```python
from build123d import *

# Parameters (mm, degrees)
SKETCH2_3_R             = 1.15
CUT_EXTRUDE1_DEPTH      = 4.9
CUT_EXTRUDE1_DEPTH_BACK = 4.9
SKETCH3_R               = 6.9
BOSS_EXTRUDE1_DEPTH     = 3


with BuildPart() as part:
    # Sketch2 → Revolve2 (revolve)
    with BuildSketch(Plane.XY):
        with BuildLine():
            Line((18.675, 0), (-12.525, 0))
            ThreePointArc((-12.525, 0), (-13.675, -1.15), (-14.825, 0))
            Line((-14.825, 0), (-18.675, 0))
            Line((-18.675, 0), (-18.675, -3.9))
            Line((-18.675, -3.9), (18.675, -3.9))
            Line((18.675, -3.9), (18.675, 0))
        make_face()
    revolve(axis=Axis((-18.675, 0, 0), (1, 0, 0)))

    # Sketch2<3> → Cut-Extrude1 (cut, two sides)
    with BuildSketch(Plane.XY) as cut_extrude1_sk:
        with Locations((-13.675, 0)):
            Circle(SKETCH2_3_R)
    extrude(amount=CUT_EXTRUDE1_DEPTH, mode=Mode.SUBTRACT)
    extrude(cut_extrude1_sk.sketch, amount=-CUT_EXTRUDE1_DEPTH_BACK, mode=Mode.SUBTRACT)

    # Sketch3 → Boss-Extrude1 (add)
    with BuildSketch(Plane(origin=(18.675, 0, 0), x_dir=(0, 0, -1), z_dir=(1, 0, 0))):
        Circle(SKETCH3_R)
    extrude(amount=BOSS_EXTRUDE1_DEPTH)


solid = part.part
```
Check sheet for the modelled part. Datum: model origin and axes. Units: mm. A direction names the side the tool comes from. Give positions to 0.01 mm unless a question says otherwise; leave off trailing zeros. Order: outer loops, then holes, each group sorted by start corner. A loop starts at its lowest first (then second) coordinate and runs counter-clockwise, first axis right, second up. Notation, with made-up numbers: (4.5, 75.5) -> (8.5, 75.5) arc R18 ccw to (8.5, 81.5) -> close; hole circle Ø6 at (36.25, -40). An arc over 180 degrees is marked (long way). Return JSON: item names as keys, results as strings.
1. Cross-section at D-D, the plane y = -2.5. Record the cut outline in (x, z) (3 decimals).
From the geometry:
{"outline": "(-18.675, -2.993) -> (18.675, -2.993) -> (18.675, -6.431) -> (21.675, -6.431) -> (21.675, 6.431) -> (18.675, 6.431) -> (18.675, 2.993) -> (-18.675, 2.993) -> close"}
2. Go/stop test with flat-tipped pins: P1, Ø3, axis at x = -13.5, y = 5.5, coming from the -Z side; P2, Ø6, axis at x = -7, y = -2.5, coming from the -Z side; P3, Ø1, axis at x = -5.5, y = -3, coming from the -Z side. Record where each tip stops, or that it passes through.
From the geometry:
{"P1": "through", "P2": "z = -3.9", "P3": "z = -2.99"}
3. Material ranges on probe 1 along X at (y, z) = (0, 1) (3 decimals); probe 2 along X at (y, z) = (-4.5, -2.5) (3 decimals); probe 3 along Z at (x, y) = (11, 0), recorded low to high. Write a range as [from, to].
From the geometry:
{"probe 1": "[-18.675, -14.825], [-12.525, 21.675]", "probe 2": "[18.675, 21.675]", "probe 3": "[-3.9, 3.9]"}
4. Set-up check for faces 1 (the flat face through (18.675, -3, -3)), 2 (the flat face through (21.675, 0, 0)): record each of +Z, -Z, +X, -X, +Y, -Y from which the full face is reachable in a straight line by a thin tool's end or side.
From the geometry:
{"face 1": "-X", "face 2": "+Z, -Z, +X, +Y, -Y"}
5. Cross-section at B-B, the plane z = 0. Record the cut outline in (x, y) (3 decimals), plus the area to 3 significant figures.
From the geometry:
{"outline": "(-18.675, -3.9) -> (18.675, -3.9) -> (18.675, -6.9) -> (21.675, -6.9) -> (21.675, 6.9) -> (18.675, 6.9) -> (18.675, 3.9) -> (-18.675, 3.9) -> close; hole circle Ø2.3 at (-13.675, 0)", "area": "329 mm^2"}
6. Cross-section at A-A, the plane y = 0. Record the cut outline in (x, z) (3 decimals), plus the area to 3 significant figures.
From the geometry:
{"outline": "(-18.675, -3.9) -> (-14.825, -3.9) -> (-14.825, 3.9) -> (-18.675, 3.9) -> close; (-12.525, -3.9) -> (18.675, -3.9) -> (18.675, -6.9) -> (21.675, -6.9) -> (21.675, 6.9) -> (18.675, 6.9) -> (18.675, 3.9) -> (-12.525, 3.9) -> close", "area": "315 mm^2"}
7. Cross-section at C-C, the plane x = -14. Record the cut outline in (y, z).
From the geometry:
{"outline": "(-1.1, -3.74) -> (-1.1, 3.74) arc R3.9 ccw to start; (1.1, -3.74) arc R3.9 ccw to (1.1, 3.74) -> close"}
